Model file for the job. Use its own axes, mm. A direction names the side the tool comes from. Give positions to 0.01 mm unless a question says otherwise; leave off trailing zeros. Write each loop counter-clockwise with the first axis right and the second up, starting at its lowest first coordinate (ties: lowest second). Pieces come first, ordered by that corner, then holes.
```python
from build123d import *

# Parameters (mm, degrees)
F0_R     = 10.925
F1_DEPTH = 8


with BuildPart() as f1:
    # F0 (on Front) → F1 (new body)
    with BuildSketch(Plane.XZ):
        with BuildLine():
            Line((-225.7977879047, -8.6602540378), (-225.7977879047, -12.5))
            Line((-225.7977879047, -12.5), (-232.4484229994, -12.5))
            Line((-232.4484229994, -12.5), (-240.7977879047, -17.3205080757))
            Line((-240.7977879047, -17.3205080757), (-215.8218352628, -31.7403810568))
            ThreePointArc((-215.8218352628, -31.7403810568), (-212.0277400373, -32.2398831693), (-208.9917082439, -29.9102540378))
            Line((-208.9917082439, -29.9102540378), (-198.9917082439, -12.5897459622))
            ThreePointArc((-198.9917082439, -12.5897459622), (-198.4922061314, -8.7956507366), (-200.8218352628, -5.7596189432))
            Line((-200.8218352628, -5.7596189432), (-225.7977879047, 8.6602540378))
            Line((-225.7977879047, 8.6602540378), (-225.7977879047, -0.9807621135))
            Line((-225.7977879047, -0.9807621135), (-222.4724703574, -6.7403810568))
            Line((-222.4724703574, -6.7403810568), (-225.7977879047, -8.6602540378))
        make_face()
        with Locations((-214.8170257912, -15)):
            Circle(F0_R, mode=Mode.SUBTRACT)
        Polygon((-240.7977879047, -17.3205080757), (-232.4484229994, -12.5), (-249.1471528101, -12.5), align=None)
        with BuildLine():
            Line((-240.7977879047, -17.3205080757), (-249.1471528101, -12.5))
            Line((-249.1471528101, -12.5), (-255.7977879047, -12.5))
            Line((-255.7977879047, -12.5), (-255.7977879047, -8.6602540378))
            Line((-255.7977879047, -8.6602540378), (-259.123105452, -6.7403810568))
            Line((-259.123105452, -6.7403810568), (-255.7977879047, -0.9807621135))
            Line((-255.7977879047, -0.9807621135), (-255.7977879047, 8.6602540378))
            Line((-255.7977879047, 8.6602540378), (-280.7737405467, -5.7596189432))
            ThreePointArc((-280.7737405467, -5.7596189432), (-283.1033696781, -8.7956507366), (-282.6038675656, -12.5897459622))
            Line((-282.6038675656, -12.5897459622), (-272.6038675656, -29.9102540378))
            ThreePointArc((-272.6038675656, -29.9102540378), (-269.5678357722, -32.2398831693), (-265.7737405467, -31.7403810568))
            Line((-265.7737405467, -31.7403810568), (-240.7977879047, -17.3205080757))
        make_face()
        with Locations((-266.7785500183, -15)):
            Circle(F0_R, mode=Mode.SUBTRACT)
        Polygon((-234.1471528101, 13.4807621135), (-225.7977879047, -0.9807621135), (-225.7977879047, 8.6602540378), align=None)
        with BuildLine():
            Line((-234.1471528101, 13.4807621135), (-225.7977879047, 8.6602540378))
            Line((-225.7977879047, 8.6602540378), (-225.7977879047, 37.5))
            ThreePointArc((-225.7977879047, 37.5), (-227.2622539988, 41.0355339059), (-230.7977879047, 42.5))
            Line((-230.7977879047, 42.5), (-250.7977879047, 42.5))
            ThreePointArc((-250.7977879047, 42.5), (-254.3333218107, 41.0355339059), (-255.7977879047, 37.5))
            Line((-255.7977879047, 37.5), (-255.7977879047, 8.6602540378))
            Line((-255.7977879047, 8.6602540378), (-247.4484229994, 13.4807621135))
            Line((-247.4484229994, 13.4807621135), (-244.123105452, 19.2403810568))
            Line((-244.123105452, 19.2403810568), (-240.7977879047, 17.3205080757))
            Line((-240.7977879047, 17.3205080757), (-237.4724703574, 19.2403810568))
            Line((-237.4724703574, 19.2403810568), (-234.1471528101, 13.4807621135))
        make_face()
        with Locations((-240.7977879047, 30)):
            Circle(F0_R, mode=Mode.SUBTRACT)
        Polygon((-255.7977879047, 8.6602540378), (-255.7977879047, -0.9807621135), (-247.4484229994, 13.4807621135), align=None)
        Polygon((-247.4484229994, 13.4807621135), (-240.7977879047, 17.3205080757), (-244.123105452, 19.2403810568), align=None)
        Polygon((-240.7977879047, 17.3205080757), (-234.1471528101, 13.4807621135), (-237.4724703574, 19.2403810568), align=None)
        Polygon((-249.1471528101, -12.5), (-232.4484229994, -12.5), (-225.7977879047, -8.6602540378), (-225.7977879047, -0.9807621135), (-234.1471528101, 13.4807621135), (-240.7977879047, 17.3205080757), (-247.4484229994, 13.4807621135), (-255.7977879047, -0.9807621135), (-255.7977879047, -8.6602540378), align=None)
        with Locations((-240.7977879047, 0)):
            Circle(F0_R, mode=Mode.SUBTRACT)
        Polygon((-225.7977879047, -0.9807621135), (-225.7977879047, -8.6602540378), (-222.4724703574, -6.7403810568), align=None)
        Polygon((-232.4484229994, -12.5), (-225.7977879047, -12.5), (-225.7977879047, -8.6602540378), align=None)
        Polygon((-255.7977879047, -12.5), (-249.1471528101, -12.5), (-255.7977879047, -8.6602540378), align=None)
        Polygon((-259.123105452, -6.7403810568), (-255.7977879047, -8.6602540378), (-255.7977879047, -0.9807621135), align=None)
    extrude(amount=F1_DEPTH)


solid = f1.part
```
1. Which spindle directions (+Z, -Z, +X, -X, +Y, -Y) get a long thin tool onto all of the face, cutting with end or side? Do faces 1 (the flat face through (-241, -4, 42.5)), 2 (the flat face through (-238, -8, -11)), 3 (the flat face through (-225.798, -4, 23)), 4 (the flat face through (-255.798, -4, 23)), 5 (the flat face through (-253.46, -3.94, -24.63)). Say none if no direction does.
Calculated:
face 1: +Z, +X, -X, +Y, -Y
face 2: +Z, -Z, +X, -X, -Y
face 3: +Z, +X, +Y, -Y
face 4: +Z, -X, +Y, -Y
face 5: -Z, +Y, -Y
2. Slice it at B-B, the plane z = -9. Write the cut outline in (x, y).
Calculated:
outline: (-283.15, -8) - (-275.91, -8) - (-275.91, 0) - (-283.15, 0) - close; (-257.65, -8) - (-246.99, -8) - (-246.99, 0) - (-257.65, 0) - close; (-234.6, -8) - (-223.95, -8) - (-223.95, 0) - (-234.6, 0) - close; (-205.69, -8) - (-198.44, -8) - (-198.44, 0) - (-205.69, 0) - close
3. Probe probe 1 along Z at (x, y) = (-250.5, -2.5); probe 2 along Z at (x, y) = (-241.5, -3.5); probe 3 along X at (y, z) = (-7.5, 16). List the from-to ranges inside material, lowest first.
Calculated:
probe 1: z = -22.92 to -5.02, 5.02 to 24.98, 35.02 to 42.5
probe 2: z = -17.73 to -10.9, 10.9 to 19.1, 40.9 to 42.5
probe 3: x = -255.8 to -225.8
4. Pin check, flat tips, straight feed: P1, Ø2, axis at y = -7, z = 26.5, coming from the -X side; P2, Ø2, axis at x = -213, y = -1.5, coming from the +Z side; P3, Ø4, axis at x = -223.5, y = -4.5, coming from the -Z side; P4, Ø4, axis at y = -1.5, z = -9, coming from the -X side. Stop position of each tip, or through.
Calculated:
P1: stops at x = -255.8
P2: stops at z = 1.85
P3: stops at z = -28.46
P4: stops at x = -283.27
5. Slice it at C-C, the plane y = -2.25. State how many separate pieces and enclosed holes the cut face has, and give its area (3 significant figures).
Calculated:
separate pieces: 1
enclosed holes: 4
area: 1,900 mm2
6. Slice it at D-D, the plane x = -214.5. Write the cut outline in (y, z), and give its area (3 significant figures).
Calculated:
outline: (-8, -32.27) - (0, -32.27) - (0, -25.92) - (-8, -25.92) - close; (-8, -4.08) - (0, -4.08) - (0, 2.14) - (-8, 2.14) - close
area: 101 mm2
7. Slice it at A-A, the plane z = 30. Write the cut outline in (x, y).
Calculated:
outline: (-255.8, -8) - (-251.72, -8) - (-251.72, 0) - (-255.8, 0) - close; (-229.87, -8) - (-225.8, -8) - (-225.8, 0) - (-229.87, 0) - close
8. Pull direction Z, two halves, no side cores. Call faces 6 (the cylindrical face through (-235.757, -3.944, -9.692)), 7 (the flat face through (-277.674, -3.944, -21.129)), 8 (the cylindrical face through (-198.48, -3.94, -8.85)): +Z half, -Z half, draft (parallel to the pull), parting line (faces both ways), or undercut.
Calculated:
face 6: undercut
face 7: -Z half
face 8: parting line
